Geometry check sheet. Reference: drawing and pictorial views, mm from the part's lowest x, y, z. A direction names the side the tool comes from. Coordinates: 2 decimals unless noted, no trailing zeros. Loops run counter-clockwise (first coordinate to the right, second up) from the corner with the lowest first, then second, coordinate; pieces in that order, holes last. Notation, with made-up numbers: (19.25, 15.5) -> (32.25, 15.5) arc R19 ccw to (32.25, 24.5) -> close; hole circle Ø5 at (-38.75, 64). An arc over 180 degrees is marked (long way). Use one line per item in the form item = value.
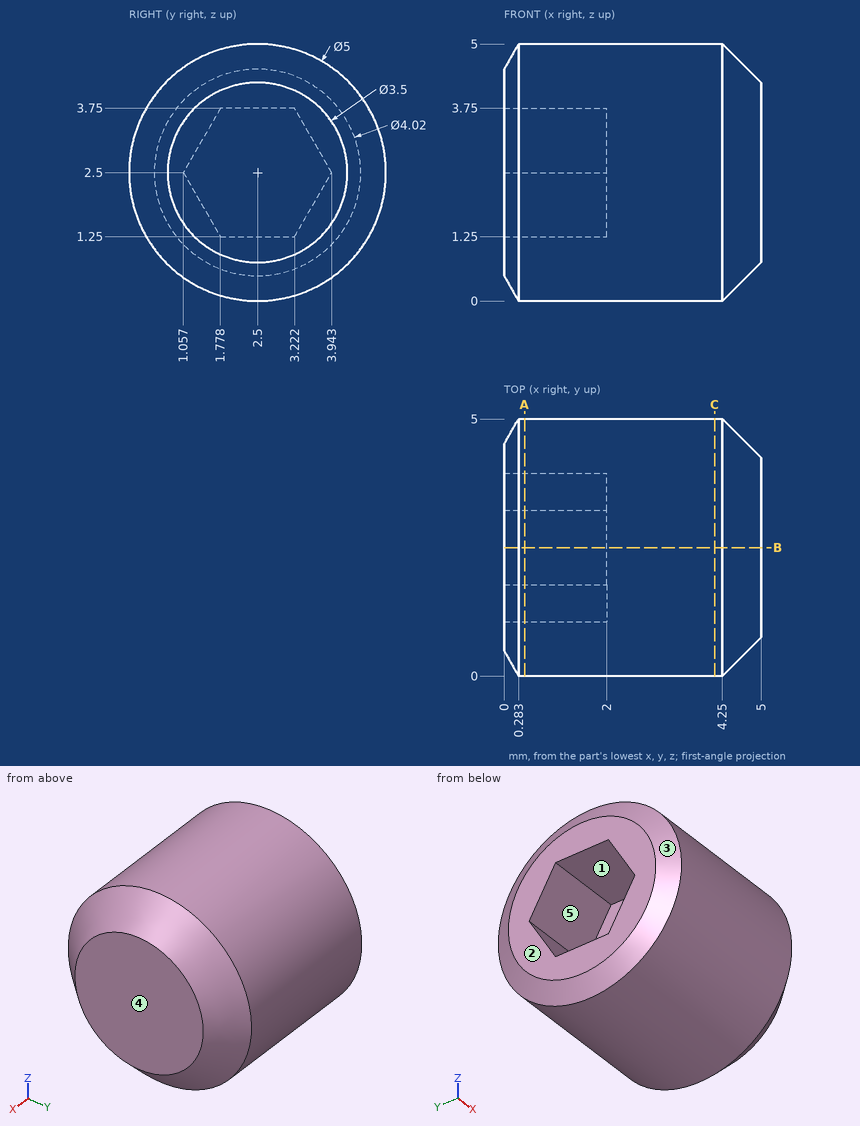
(1) Section check A-A, the plane x = 0.4. Record the boundary of the cut face in (y, z), plus the area to 3 significant figures.
Established:
outline = circle Ø5 at (2.5, 2.5); hole (1.06, 2.5) -> (1.78, 1.25) -> (3.22, 1.25) -> (3.94, 2.5) -> (3.22, 3.75) -> (1.78, 3.75) -> close
area = 14.2 mm²
(2) Tool access check on the marked faces 4 and 5. Record the directions out of +Z, -Z, +X, -X, +Y, -Y that give a thin tool (end or side, any length) a straight path to the whole face; none if there is none.
Established:
face_4 = +Z, -Z, +X, +Y, -Y
face_5 = -X
(3) Go/stop test with a flat-tipped pin: P1, Ø3, axis at y = 2.5, z = 2, coming from the -X side. Record where the tip stops, or that it passes through.
Established:
P1 = 0
(4) Section check B-B, the plane y = 2.5. Record the boundary of the cut face in (x, z), plus the area to 3 significant figures.
Established:
outline = (0, 0.49) -> (0.28, 0) -> (4.25, 0) -> (5, 0.75) -> (5, 4.25) -> (4.25, 5) -> (0.28, 5) -> (0, 4.51) -> (0, 3.75) -> (2, 3.75) -> (2, 1.25) -> (0, 1.25) -> close
area = 19.3 mm²
(5) Mould release check, pull along Y, two halves, no side actions. Record for the marked faces 1, 2 and 3: +Y half, -Y half, draft (parallel to the pull), parting line (faces both ways), or undercut.
Established:
face_1 = undercut
face_2 = draft
face_3 = parting line
(6) Scan lines: line 1 along X through (y, z) = (3.05, 2.55); line 2 along Z through (x, y) = (1.95, 3.55); line 3 along Z through (x, y) = (0.8, 2.75). Record each from-to range of solid material in increasing order.
Established:
line_1 = 2 to 5
line_2 = 0.23 to 1.82, 3.18 to 4.77
line_3 = 0.01 to 1.25, 3.75 to 4.99
(7) Section check C-C, the plane x = 4.1. Record the boundary of the cut face in (y, z).
Established:
outline = circle Ø5 at (2.5, 2.5)
